from build123d import *

# Parameters (mm, degrees)
F0_W     = 100
F0_H     = 100
F1_DEPTH = 20
F3_D     = 8.5
F5_D     = 13
F6_R     = 10


with BuildPart() as f1:
    # F0 (on Top) → F1 (new body)
    with BuildSketch(Plane.XY):
        Rectangle(F0_W, F0_H)
    extrude(amount=F1_DEPTH)

    # F3 (through all)
    with Locations(Plane.XZ.offset(50)):
        with Locations((0, 10.0764958188)):
            Hole(F3_D / 2)

    # F5 (through all)
    with Locations(Plane.XY.offset(20)):
        with Locations((0, 0)):
            Hole(F5_D / 2)

    # F6
    f6_edges = [f1.edges().sort_by_distance(p)[0] for p in [
        (50, -50, 10),
        (-50, -50, 10),
        (50, 50, 10),
        (-50, 50, 10),
    ]]
    fillet(f6_edges, radius=F6_R)


solid = f1.part
Build history of the part. All positions in model axes, mm. Give positions to 0.01 mm unless a question says otherwise; leave off trailing zeros. Write each loop counter-clockwise with the first axis right and the second up, starting at its lowest first coordinate (ties: lowest second). Pieces come first, ordered by that corner, then holes. Notation, with made-up numbers: (27.5, 17.5) - (46.5, 17.5) arc R29 cw to (46.5, 37.5) - close; hole circle Ø10 at (23.5, 80). An arc over 180 degrees is marked (long way). Use one line per item in the form item = value. Start each with the question number.
1. Band-saw the part on B-B on y = 0. Write the cut outline in (x, z).
2. Band-saw the part on D-D on y = 32.5. Write the cut outline in (x, z), plus the area to 3 significant figures.
3. Band-saw the part on A-A on x = 0. Write the cut outline in (y, z).
4. Probe line 1 (Z direction, x = 0, y = 30.5); line 2 (X direction, y = 36, z = 10.5); line 3 (Y direction, x = 0, z = 4.75). List the from-to ranges inside material, lowest first. Write a range as [from, to].
5. Two-plate mould, pull along Z, no slides. Class faces 1 (the face through (0.921, -27.143, 5.928)), 2 (the face through (-1, 50, 5)), 3 (the face through (-1, 12, 20)): released by +Z, released by -Z, zero draft, split by the parting line, or undercut.
6. Drop a flat-ended pin along its axis: pin 1 Ø11 at (x, z) = (0, 10.08) entering from -Y. Give the stop position or say it passes through.
7. Band-saw the part on C-C on z = 4. Write the cut outline in (x, y), plus the area to 3 significant figures.
Conclusion:
q1.outline = (-50, 0) - (-6.5, 0) - (-6.5, 20) - (-50, 20) - close; (6.5, 0) - (50, 0) - (50, 20) - (6.5, 20) - close
q2.outline = (-50, 0) - (50, 0) - (50, 20) - (-50, 20) - close; hole circle Ø8.5 at (0, 10.08)
q2.area = 1,940 mm²
q3.outline = (-50, 0) - (-6.5, 0) - (-6.5, 5.83) - (-50, 5.83) - close; (-50, 14.33) - (-6.5, 14.33) - (-6.5, 20) - (-50, 20) - close; (6.5, 0) - (50, 0) - (50, 5.83) - (6.5, 5.83) - close; (6.5, 14.33) - (50, 14.33) - (50, 20) - (6.5, 20) - close
q4.line_1 = [0, 5.83], [14.33, 20]
q4.line_2 = [-50, -4.23], [4.23, 50]
q4.line_3 = [-50, -6.5], [6.5, 50]
q5.face_1 = undercut
q5.face_2 = zero draft
q5.face_3 = released by +Z
q6.pin_1 = -50
q7.outline = (-50, -40) arc R10 ccw to (-40, -50) - (40, -50) arc R10 ccw to (50, -40) - (50, 40) arc R10 ccw to (40, 50) - (-40, 50) arc R10 ccw to (-50, 40) - close; hole circle Ø13 at (0, 0)
q7.area = 9,780 mm²
